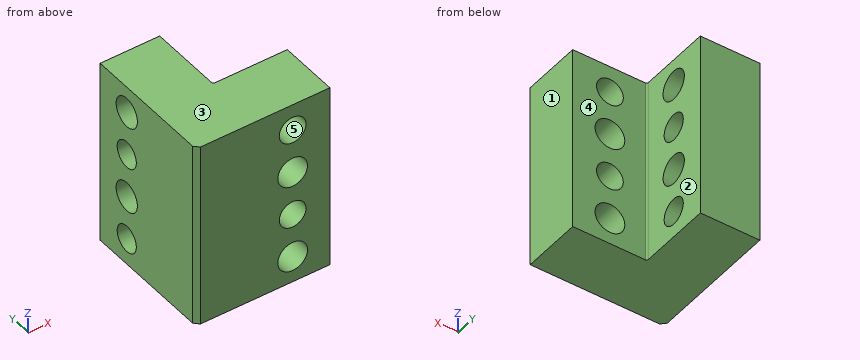
```python
from build123d import *

# Parameters (mm, degrees)
F1_DEPTH = 63
F2_R     = 4.5
F2_R_2   = 5
F3_DEPTH = 25
F4_R     = 4.5
F4_R_2   = 5
F5_DEPTH = 25
F6_R     = 0.5
F7_SIZE  = 1.5


with BuildPart() as f1:
    # F0 (on Top) → F1 (new body)
    with BuildSketch(Plane.XY):
        Polygon((-45, 0), (0, 0), (0, 20), (-25, 20), (-25, 45), (-45, 45), align=None)
    extrude(amount=F1_DEPTH)

    # F2 (on face) → F3 (cut)
    with BuildSketch(Plane.YZ.offset(-25)):
        with Locations((32.5, 39)):
            Circle(F2_R)
        with Locations((32.5, 24)):
            Circle(F2_R_2)
        with Locations((32.5, 9)):
            Circle(F2_R)
        with Locations((32.5, 54)):
            Circle(F2_R_2)
    extrude(amount=-F3_DEPTH, mode=Mode.SUBTRACT)

    # F4 (on face) → F5 (cut)
    with BuildSketch(Plane(origin=(0, 20, 0), x_dir=(-1, 0, 0), z_dir=(0, 1, 0))):
        with Locations((12.5, 54)):
            Circle(F4_R)
        with Locations((12.5, 39)):
            Circle(F4_R_2)
        with Locations((12.5, 24)):
            Circle(F4_R)
        with Locations((12.5, 9)):
            Circle(F4_R_2)
    extrude(amount=-F5_DEPTH, mode=Mode.SUBTRACT)

    # F6
    f6_edges = [f1.edges().sort_by_distance(p)[0] for p in [
        (-25, 20, 31.5),
    ]]
    fillet(f6_edges, radius=F6_R)

    # F7
    f7_edges = [f1.edges().sort_by_distance(p)[0] for p in [
        (-45, 0, 31.5),
    ]]
    chamfer(f7_edges, length=F7_SIZE)


solid = f1.part
```
The model under review builds one solid part; all positions refer to its coordinate system, in mm. Face numbers are marked on the shaded views. A direction names the side the tool comes from. Round coordinates to 2 decimals unless told otherwise and drop trailing zeros. Loops run counter-clockwise (first coordinate to the right, second up) from the corner with the lowest first, then second, coordinate; pieces in that order, holes last.
Item 1: Clearance check with flat-ended pins moving along their axes: pin 1 Ø10.5 at (y, z) = (32.5, 9) entering from +X; pin 2 Ø7 at (x, z) = (-12.5, 54) entering from +Y; pin 3 Ø8 at (x, z) = (-9, 48.5) entering from +Y. State where each tip first meets the part, or that it passes through.
Determined:
pin 1: stops at x = -25
pin 2: passes through
pin 3: stops at y = 20
Item 2: Take a section at B-B (y = 6.5). Write out the cut boundary in (x, z).
Determined:
outline: (-45, 0) - (0, 0) - (0, 63) - (-45, 63) - close; hole circle Ø10 at (-12.5, 9); hole circle Ø10 at (-12.5, 39); hole circle Ø9 at (-12.5, 24); hole circle Ø9 at (-12.5, 54)
Item 3: Take a section at C-C (x = -30). Write out the cut boundary in (y, z), then the cut area to 3 significant figures.
Determined:
outline: (0, 0) - (45, 0) - (45, 63) - (0, 63) - close; hole circle Ø10 at (32.5, 24); hole circle Ø10 at (32.5, 54); hole circle Ø9 at (32.5, 9); hole circle Ø9 at (32.5, 39)
area: 2,550 mm2
Item 4: For the marked faces 1 and 2, list the 3-axis set-ups (+Z, -Z, +X, -X, +Y, -Y) from which the entire face can be reached by the end or side of a thin tool; tool diameter is ignored.
Determined:
face 1: +Z, -Z, +X, +Y, -Y
face 2: +Z, -Z, +X, +Y
Item 5: Take a section at D-D (z = 45). Write out the cut boundary in (x, y), then the cut area to 3 significant figures.
Determined:
outline: (-45, 1.5) - (-43.5, 0) - (0, 0) - (0, 20) - (-24.5, 20) arc R0.5 cw to (-25, 20.5) - (-25, 45) - (-45, 45) - close
area: 1,400 mm2
Item 6: Take a section at A-A (z = 24). Write out the cut boundary in (x, y).
Determined:
outline: (-45, 1.5) - (-43.5, 0) - (-17, 0) - (-17, 20) - (-24.5, 20) arc R0.5 cw to (-25, 20.5) - (-25, 27.5) - (-45, 27.5) - close; (-45, 37.5) - (-25, 37.5) - (-25, 45) - (-45, 45) - close; (-8, 0) - (0, 0) - (0, 20) - (-8, 20) - close
Item 7: For line 1 (Z direction, x = -12.5, y = 15); line 2 (Y direction, x = -7, z = 3); line 3 (X direction, y = 37, z = 8), list the stretches that pass through material, from the lowest coordinate up.
Determined:
line 1: z = 0 to 4, 14 to 19.5, 28.5 to 34, 44 to 49.5, 58.5 to 63
line 2: y = 0 to 20
line 3: x = -45 to -25
Item 8: Mouldability with a two-part tool opening along Z and no side actions: class the marked faces 3, 4 and 5 as released by +Z, released by -Z, zero draft, split by the parting line, or undercut.
Determined:
face 3: released by +Z
face 4: zero draft
face 5: undercut
